For this review, take the finished solid that the model builds, in its own axes (mm). A direction names the side the tool comes from. Give positions to 0.01 mm unless a question says otherwise; leave off trailing zeros. Write each loop counter-clockwise with the first axis right and the second up, starting at its lowest first coordinate (ties: lowest second). Pieces come first, ordered by that corner, then holes.
from build123d import *

# Parameters (mm, degrees)
SKETCH1_R           = 4
BOSS_EXTRUDE1_DEPTH = 10


with BuildPart() as part:
    # Sketch1 → Boss-Extrude1 (new body)
    with BuildSketch(Plane(origin=(0, 0, 0), x_dir=(1, 0, 0), z_dir=(0, 1, 0))):
        with BuildLine():
            Line((0, 0), (40, 0))
            Line((40, 0), (68.284271247, 28.284271247))
            Line((68.284271247, 28.284271247), (108.284271247, 28.284271247))
            ThreePointArc((108.284271247, 28.284271247), (133.284271247, 53.284271247), (108.284271247, 78.284271247))
            Line((108.284271247, 78.284271247), (68.284271247, 78.284271247))
            Line((68.284271247, 78.284271247), (32.928932188, 113.639610307))
            Line((32.928932188, 113.639610307), (7.071067812, 113.639610307))
            Line((7.071067812, 113.639610307), (-28.284271247, 78.284271247))
            Line((-28.284271247, 78.284271247), (-28.284271247, 28.284271247))
            Line((-28.284271247, 28.284271247), (0, 0))
        make_face()
        with Locations(Location((5, 100, 0), (0, 0, 270))):
            Circle(SKETCH1_R, mode=Mode.SUBTRACT)
        with Locations(Location((35, 100, 0), (0, 0, 270))):
            Circle(SKETCH1_R, mode=Mode.SUBTRACT)
        with Locations(Location((-13.284271247, 53.284271247, 0), (0, 0, 270))):
            Circle(SKETCH1_R, mode=Mode.SUBTRACT)
        with BuildLine():
            Line((53.284271247, 68.284271247), (83.284271247, 68.284271247))
            ThreePointArc((83.284271247, 68.284271247), (98.284271247, 53.284271247), (83.284271247, 38.284271247))
            Line((83.284271247, 38.284271247), (53.284271247, 38.284271247))
            ThreePointArc((53.284271247, 38.284271247), (38.284271247, 53.284271247), (53.284271247, 68.284271247))
        make_face(mode=Mode.SUBTRACT)
    extrude(amount=BOSS_EXTRUDE1_DEPTH)


solid = part.part
(1) The part is to be moulded in two halves that separate along X. For faces 6 (the flat face through (68, 5, -38.284)), 7 (the cylindrical face through (133.28, 4.93, -52.73)), 8 (the flat face through (20, 5, -113.64)), say which applies: +X half, -X half, draft (parallel to the pull), parting line (faces both ways), or undercut.
(2) For L1, parallel to X at y = 9, z = -55.5; L2, parallel to X at y = 8.75, z = -50; L3, parallel to Z at x = 47, y = 7.25, list the stretches that pass through material, from the lowest coordinate up.
(3) We need section A-A (x = 75.5). Write out the cut boundary in (y, z), and give its area (3 significant figures).
(4) We need section D-D (z = -100). Write out the cut boundary in (x, y), and give its area (3 significant figures).
(5) We need section C-C (y = 6.25). Write out the cut boundary in (x, z).
(6) Clearance check with flat-ended pins moving along their axes: pin 1 Ø7 at (x, z) = (35, -100) entering from -Y; pin 2 Ø3 at (x, y) = (69, 5.5) entering from -Z; pin 3 Ø3 at (x, y) = (65.5, 5) entering from -Z; pin 4 Ø5 at (y, z) = (4, -101) entering from -X. State where each tip first meets the part, or that it passes through.
(7) We need section B-B (z = -66). Write out the cut boundary in (x, y).
(8) Tool access review of faces 1 (the flat face through (33, 0, -58)), 2 (the flat face through (89, 5, -78.284)), 3 (the cylindrical face through (98.28, 4.93, -53.61)), 4 (the flat face through (88, 5, -28.284)), 5 (the flat face through (-28.284, 5, -54)): name each direction out of +Z, -Z, +X, -X, +Y, -Y from which nothing blocks a thin tool from reaching the whole face with its end or side.
The answers:
1. face 6: undercut
1. face 7: +X half
1. face 8: draft
2. L1: x = -28.28 to -16.61, -9.95 to 38.45, 98.12 to 133.19
2. L2: x = -28.28 to -15.57, -11 to 38.65, 97.92 to 133.07
2. L3: z = -99.57 to -66.9, -39.66 to -7
3. outline: (0, -78.28) - (10, -78.28) - (10, -68.28) - (0, -68.28) - close; (0, -38.28) - (10, -38.28) - (10, -28.28) - (0, -28.28) - close
3. area: 200 mm2
4. outline: (-6.57, 0) - (1, 0) - (1, 10) - (-6.57, 10) - close; (9, 0) - (31, 0) - (31, 10) - (9, 10) - close; (39, 0) - (46.57, 0) - (46.57, 10) - (39, 10) - close
4. area: 371 mm2
5. outline: (-28.28, -78.28) - (7.07, -113.64) - (32.93, -113.64) - (68.28, -78.28) - (108.28, -78.28) arc R25 ccw to (108.28, -28.28) - (68.28, -28.28) - (40, 0) - (0, 0) - (-28.28, -28.28) - close; hole circle Ø8 at (-13.28, -53.28); hole circle Ø8 at (5, -100); hole circle Ø8 at (35, -100); hole (53.28, -68.28) - (83.28, -68.28) arc R15 ccw to (83.28, -38.28) - (53.28, -38.28) arc R15 ccw to start
6. pin 1: passes through
6. pin 2: stops at z = -79.07
6. pin 3: stops at z = -82.57
6. pin 4: stops at x = -8.07
7. outline: (-28.28, 0) - (45.33, 0) - (45.33, 10) - (-28.28, 10) - close; (91.24, 0) - (129.81, 0) - (129.81, 10) - (91.24, 10) - close
8. face 1: +Z, -Z, +X, -X, -Y
8. face 2: -Z, +X, +Y, -Y
8. face 3: +Y, -Y
8. face 4: +Z, +X, +Y, -Y
8. face 5: +Z, -Z, -X, +Y, -Y
